from build123d import *

# Parameters (mm, degrees)
F0_R        = 5.7271899427
F0_R_2      = 6.0263161758
F0_R_3      = 5.6540098822
F0_R_4      = 5.7746792183
F1_DEPTH    = 15.24
F2_T1_DEPTH = 18.788208103
F2_T3_DEPTH = 18.873984206


# Not quite as in the source:
# - a fillet or chamfer that OpenCascade refuses, or shapes differently, is made with other operations: its cross-section is extruded or revolved along the edge and cut away or added


with BuildPart() as f1:
    # F0 (on Top) → F1 (new body)
    with BuildSketch(Plane.XY):
        with BuildLine():
            Line((-126.2685924224, 95.313180417), (-179.9737472962, 95.313180417))
            ThreePointArc((-179.9737472962, 95.313180417), (-185.2842850362, 93.1578477365), (-187.5906297205, 87.9111302629))
            Line((-187.5906297205, 87.9111302629), (-188.941179568, 40.7122925946))
            Line((-188.941179568, 40.7122925946), (-187.5906297205, -6.4865450738))
            ThreePointArc((-187.5906297205, -6.4865450738), (-185.2842850362, -11.7332625474), (-179.9737472962, -13.8885952279))
            Line((-179.9737472962, -13.8885952279), (-126.2685924224, -13.8885952279))
            ThreePointArc((-126.2685924224, -13.8885952279), (-120.9562110346, -11.7314702942), (-118.6515646464, -6.4814046742))
            Line((-118.6515646464, -6.4814046742), (-117.3330366223, 40.7122925946))
            Line((-117.3330366223, 40.7122925946), (-118.6515646464, 87.9059898633))
            ThreePointArc((-118.6515646464, 87.9059898633), (-120.9562110346, 93.1560554834), (-126.2685924224, 95.313180417))
        make_face()
        with Locations((-176.378503075, -2.5813533248)):
            Circle(F0_R, mode=Mode.SUBTRACT)
        with Locations((-130.0195976365, -2.5813533248)):
            Circle(F0_R_2, mode=Mode.SUBTRACT)
        with BuildLine():
            Line((-130.635044248, 59.1215779044), (-130.6350442799, 22.2915779044))
            ThreePointArc((-130.6350442799, 22.2915779044), (-133.610839383, 15.1073730075), (-140.7950442799, 12.1315779044))
            Line((-140.7950442799, 12.1315779044), (-164.9250442799, 12.1315779044))
            ThreePointArc((-164.9250442799, 12.1315779044), (-172.1092491767, 15.1073730075), (-175.0850442799, 22.2915779044))
            Line((-175.0850442799, 22.2915779044), (-175.0850442799, 59.1215779044))
            ThreePointArc((-175.0850442799, 59.1215779044), (-172.1092491767, 66.3057828012), (-164.9250442799, 69.2815779044))
            Line((-164.9250442799, 69.2815779044), (-140.7950442799, 69.2815779044))
            ThreePointArc((-140.7950442799, 69.2815779044), (-133.6108393717, 66.3057828031), (-130.635044248, 59.1215779044))
        make_face(mode=Mode.SUBTRACT)
        with Locations((-176.378503075, 84.005938514)):
            Circle(F0_R_3, mode=Mode.SUBTRACT)
        with Locations((-130.0195976365, 84.005938514)):
            Circle(F0_R_4, mode=Mode.SUBTRACT)
    extrude(amount=F1_DEPTH)

    # F2: fillet of radius 25.4 on 2 edges, made by hand

    # F2_s2 → F2_t1 (cut)
    with BuildSketch(Plane.XY.offset(-1.7741040515)):
        with BuildLine():
            ThreePointArc((-117.3528553153, 40.0029277737), (-117.3429479018, 40.7122925946), (-117.3528553153, 41.4216574155))
            Line((-117.3528553153, 41.4216574155), (-117.3330366223, 40.7122925946))
            Line((-117.3330366223, 40.7122925946), (-117.3528553153, 40.0029277737))
        make_face()
    extrude(amount=F2_T1_DEPTH, mode=Mode.SUBTRACT)

    # F2_s4 → F2_t3 (cut)
    with BuildSketch(Plane.XY.offset(-1.816992103)):
        with BuildLine():
            ThreePointArc((-188.9203914761, 41.4387920809), (-188.9307833954, 40.7122925946), (-188.9203914761, 39.9857931082))
            Line((-188.9203914761, 39.9857931082), (-188.941179568, 40.7122925946))
            Line((-188.941179568, 40.7122925946), (-188.9203914761, 41.4387920809))
        make_face()
    extrude(amount=F2_T3_DEPTH, mode=Mode.SUBTRACT)


solid = f1.part
Here's how the part is built. I have some questions about the finished solid (model axes, mm). A direction names the side the tool comes from. Round coordinates to 2 decimals unless told otherwise and drop trailing zeros. Order: outer loops, then holes, each group sorted by start corner. A loop starts at its lowest first (then second) coordinate and runs counter-clockwise, first axis right, second up. Notation, with made-up numbers: M -38.75,-37.75 L -15.75,-37.75 A37 cw -15.75,-1.75 Z; hole C 4,20.5 d1. An arc over 180 degrees is marked long. Return JSON: item names as keys, results as strings. Group by question number.
1. If we section it at B-B on y = 18.5: List the corners of the cut face in (x, z) for me.
2. If we section it at D-D on z = 11.5: List the corners of the cut face in (x, y) for me.
3. On a 3-axis mill with a long thin cutter (end or side, diameter ignored), from which of +Z, -Z, +X, -X, +Y, -Y can I reach the whole of each face in a straight line? I mean faces 1 (the face through (-153, 69.282, 8)), 2 (the face through (-130, 41, 15.24)). Say none if no direction works.
4. If we section it at A-A on x = -128.5: List the corners of the cut face in (y, z) for me.
5. If we section it at C-C on x = -161.5: List the corners of the cut face in (y, z) for me, then the cut area to 3 significant figures.
6. I'm going to push flat-ended pins straight in: pin 1 Ø7.5 at (y, z) = (49, 7.5) entering from +X; pin 2 Ø11 at (x, y) = (-130.02, -2.58) entering from -Z. Where does each tip first touch, or does it pass through?
7. If we mould it in two halves opening along X, with no side actions, what happens to faces 3 (the face through (-153, -13.889, 8)), 4 (the face through (-121.016, -11.789, 7.513)), 5 (the face through (-185.34, -11.68, 7.51)), 6 (the face through (-133.69, 66.384, 7.513))? For each: pulls with the +X half, pulls with the -X half, needs draft (parallel to the pull), parting line crosses it, or undercut.
8. Please list where these lines run through material, in increasing order: probe 1 along X at (y, z) = (89, 7.5); probe 2 along X at (y, z) = (85, 5.5); probe 3 along Y at (x, z) = (-161.5, 11.75).
Reply:
{
 "1": {"outline": "M -188.31,0 L -174.35,0 L -174.35,15.24 L -188.31,15.24 Z; M -131.37,0 L -117.95,0 L -117.95,15.24 L -131.37,15.24 Z"},
 "2": {"outline": "M -188.92,39.99 L -187.59,-6.49 A7.62 ccw -179.97,-13.89 L -126.27,-13.89 A7.62 ccw -118.65,-6.48 L -117.35,40 A25.4 ccw -117.35,41.42 L -118.65,87.91 A7.62 ccw -126.27,95.31 L -179.97,95.31 A7.62 ccw -187.59,87.91 L -188.92,41.44 A25.4 ccw Z; hole C -176.38,-2.58 d11.45; hole C -176.38,84.01 d11.31; hole M -175.09,22.29 A10.16 ccw -164.93,12.13 L -140.8,12.13 A10.16 ccw -130.64,22.29 L -130.64,59.12 A10.16 ccw -140.8,69.28 L -164.93,69.28 A10.16 ccw -175.09,59.12 Z; hole C -130.02,-2.58 d12.05; hole C -130.02,84.01 d11.55"},
 "3": {"face 1": "+Z, -Z", "face 2": "+Z, +X, -X, +Y, -Y"},
 "4": {"outline": "M -13.89,0 L -8.41,0 L -8.41,15.24 L -13.89,15.24 Z; M 3.25,0 L 78.43,0 L 78.43,15.24 L 3.25,15.24 Z; M 89.58,0 L 95.31,0 L 95.31,15.24 L 89.58,15.24 Z"},
 "5": {"outline": "M -13.89,0 L 12.13,0 L 12.13,15.24 L -13.89,15.24 Z; M 69.28,0 L 95.31,0 L 95.31,15.24 L 69.28,15.24 Z", "area": "793 mm^2"},
 "6": {"pin 1": "x = -117.46", "pin 2": "through"},
 "7": {"face 3": "needs draft", "face 4": "pulls with the +X half", "face 5": "pulls with the -X half", "face 6": "undercut"},
 "8": {"probe 1": "-187.48 to -179.03, -173.73 to -132.92, -127.12 to -118.76", "probe 2": "-187.67 to -181.94, -170.81 to -135.71, -124.33 to -118.57", "probe 3": "-13.89 to 12.13, 69.28 to 95.31"}
}
